The figure shows three views and two pictorial views of one solid part (mm, origin at its lowest corner). Answer the questions. A direction names the side the tool comes from. Coordinates: 2 decimals unless noted, no trailing zeros. Loops run counter-clockwise (first coordinate to the right, second up) from the corner with the lowest first, then second, coordinate; pieces in that order, holes last.
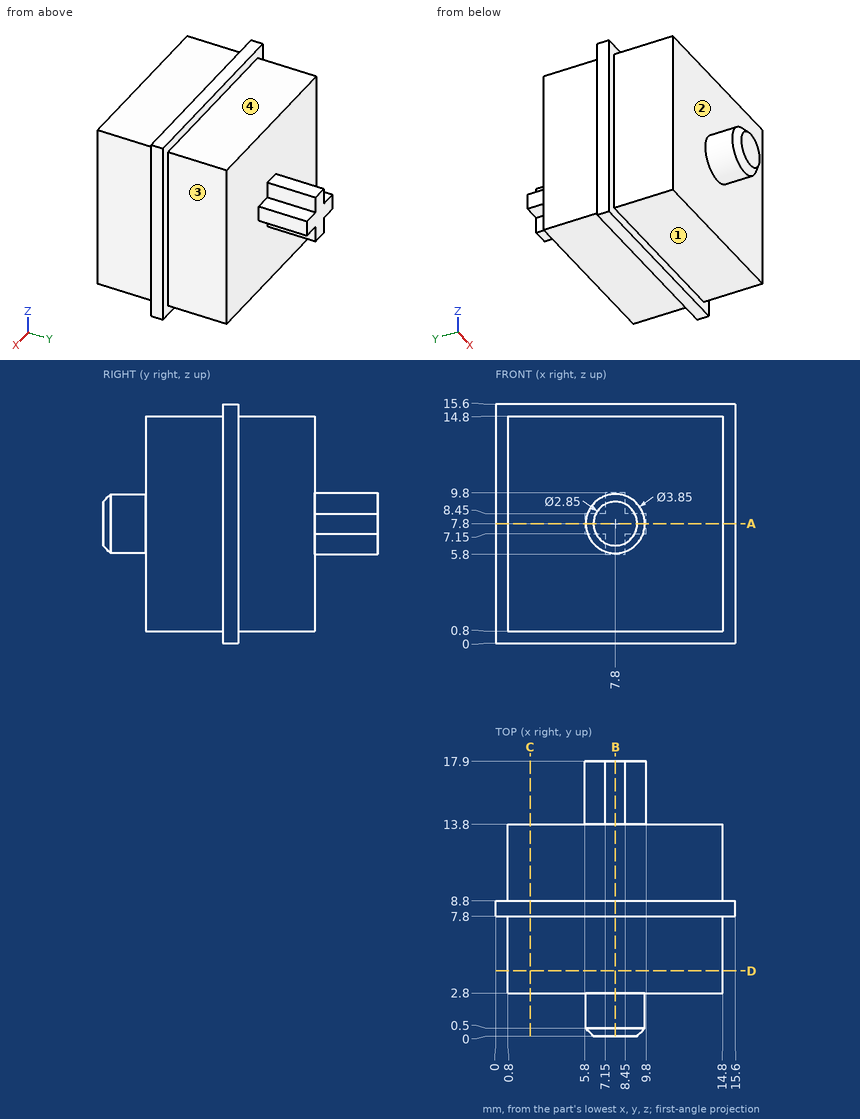
1. A cutting plane is placed at D-D, the plane y = 4.25. Give the vertices of the cut face in (x, z).
2. Straight lines are drawn through the part: probe 1 along Y at (x, z) = (13, 5.25); probe 2 along X at (y, z) = (7, 14.5); probe 3 along X at (y, z) = (15.25, 6.5). For each, find the intervals that lie inside material, in ascending order.
3. A cutting plane is placed at B-B, the plane x = 7.8. Give the vertices of the cut face in (y, z) (3 decimals), then the cut area to 3 significant figures.
4. For the marked faces 1, 2, 3 and 4, determine the directions among +Z, -Z, +X, -X, +Y, -Y from which every point of the face is accessible in a straight line to the end or side of a thin tool.
5. A cutting plane is placed at C-C, the plane x = 2.25. Give the vertices of the cut face in (y, z), then the cut area to 3 significant figures.
6. A cutting plane is placed at A-A, the plane z = 7.8. Give the vertices of the cut face in (x, y) (3 decimals).
7. Each of these flat-tipped pins is pushed along its axis until it touches: P1, Ø1.5, axis at x = 9.5, z = 2, coming from the -Y side; P2, Ø1, axis at x = 2.5, z = 6.5, coming from the +Y side; P3, Ø4, axis at y = 15.5, z = 9, coming from the -X side. Where does it stop, or does it pass through?
Answers below:
1. outline: (0.8, 0.8) - (14.8, 0.8) - (14.8, 14.8) - (0.8, 14.8) - close
2. probe 1: y = 2.8 to 13.8
2. probe 2: x = 0.8 to 14.8
2. probe 3: x = 7.15 to 8.45
3. outline: (0, 6.375) - (0.5, 5.875) - (2.8, 5.875) - (2.8, 0.8) - (7.8, 0.8) - (7.8, 0) - (8.8, 0) - (8.8, 0.8) - (13.8, 0.8) - (13.8, 5.8) - (17.9, 5.8) - (17.9, 9.8) - (13.8, 9.8) - (13.8, 14.8) - (8.8, 14.8) - (8.8, 15.6) - (7.8, 15.6) - (7.8, 14.8) - (2.8, 14.8) - (2.8, 9.725) - (0.5, 9.725) - (0, 9.225) - close
3. area: 183 mm2
4. face 1: -Z, +X, -X, -Y
4. face 2: -Y
4. face 3: +Z, -Z, +X, +Y
4. face 4: +Z, +X, -X, +Y
5. outline: (2.8, 0.8) - (7.8, 0.8) - (7.8, 0) - (8.8, 0) - (8.8, 0.8) - (13.8, 0.8) - (13.8, 14.8) - (8.8, 14.8) - (8.8, 15.6) - (7.8, 15.6) - (7.8, 14.8) - (2.8, 14.8) - close
5. area: 156 mm2
6. outline: (0, 7.8) - (0.8, 7.8) - (0.8, 2.8) - (5.875, 2.8) - (5.875, 0.5) - (6.375, 0) - (9.225, 0) - (9.725, 0.5) - (9.725, 2.8) - (14.8, 2.8) - (14.8, 7.8) - (15.6, 7.8) - (15.6, 8.8) - (14.8, 8.8) - (14.8, 13.8) - (9.8, 13.8) - (9.8, 17.9) - (5.8, 17.9) - (5.8, 13.8) - (0.8, 13.8) - (0.8, 8.8) - (0, 8.8) - close
7. P1: stops at y = 2.8
7. P2: stops at y = 13.8
7. P3: stops at x = 0.8
